For this review, take the finished solid that the model builds, in its own axes (mm). Give positions to 0.01 mm unless a question says otherwise; leave off trailing zeros. Order: outer loops, then holes, each group sorted by start corner. A loop starts at its lowest first (then second) coordinate and runs counter-clockwise, first axis right, second up. Notation, with made-up numbers: (-0.5, 64) - (37.5, 64) arc R29 cw to (37.5, 101) - close; hole circle Ø8 at (9, 18). An arc over 180 degrees is marked (long way). Use a Markdown table: item, result. Add a question column.
1) We need section C-C on y = -23. Write out the cut boundary in (x, z).
2) We need section B-B on x = 0. Write out the cut boundary in (y, z), then the cut area to 3 significant figures.
3) Wall thickness on L1, parallel to Z at x = 0, y = -22; L2, parallel to Z at x = -6, y = -4; L3, parallel to X at y = -4, z = -259.5: over which ranges is each line inside the solid? List them lowest first.
4) We need section A-A on z = 0. Write out the cut boundary in (x, y), then the cut area to 3 significant figures.
5) Clearance check with flat-ended pins moving along their axes: P1, Ø1, axis at y = -21.5, z = 223.5, coming from the -X side; P2, Ø12, axis at x = 161.5, y = -17.5, coming from the -Z side; P3, Ø2, axis at x = 233, y = -39.5, coming from the +Z side. State where each tip first meets the part, or that it passes through.
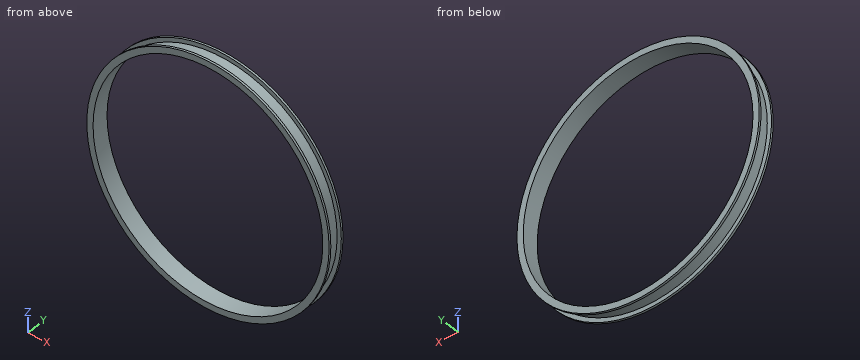
```python
from build123d import *

# Parameters (mm, degrees)
F0_R     = 368.3
F1_DEPTH = 50.8
F2_D     = 698.5
F3_T     = -6.35


with BuildPart() as f1:
    # F0 (on Front) → F1 (new body)
    with BuildSketch(Plane.XZ):
        Circle(F0_R)
    extrude(amount=F1_DEPTH)

    # F2 (through all)
    with Locations(Plane(origin=(0, 0, 0), x_dir=(1, 0, 0), z_dir=(0, 1, 0))):
        with Locations((0, 0)):
            Hole(F2_D / 2)

    # F3
    f3_openings = [f1.faces().sort_by_distance(p)[0] for p in [
        (-368.3, -25.4, 0),
    ]]
    offset(amount=F3_T, openings=f3_openings)


solid = f1.part
```
Checked values:
| question | item | result |
|---|---|---|
| 1 | outline | circle Ø711.2 at (0, 0); hole circle Ø698.5 at (0, 0) |
| 2 | outline | (-50.8, -368.3) - (-44.45, -368.3) - (-44.45, -355.6) - (-6.35, -355.6) - (-6.35, -368.3) - (0, -368.3) - (0, -349.25) - (-50.8, -349.25) - close; (-50.8, 349.25) - (0, 349.25) - (0, 368.3) - (-6.35, 368.3) - (-6.35, 355.6) - (-44.45, 355.6) - (-44.45, 368.3) - (-50.8, 368.3) - close |
| 2 | area | 968 mm² |
| 3 | L1 | -355.6 to -349.25, 349.25 to 355.6 |
| 3 | L2 | -368.25 to -349.2, 349.2 to 368.25 |
| 3 | L3 | -261.35 to -233.74, 233.74 to 261.35 |
| 4 | outline | (-368.3, -50.8) - (-349.25, -50.8) - (-349.25, 0) - (-368.3, 0) - (-368.3, -6.35) - (-355.6, -6.35) - (-355.6, -44.45) - (-368.3, -44.45) - close; (349.25, -50.8) - (368.3, -50.8) - (368.3, -44.45) - (355.6, -44.45) - (355.6, -6.35) - (368.3, -6.35) - (368.3, 0) - (349.25, 0) - close |
| 4 | area | 968 mm² |
| 5 | P1 | x = -276.99 |
| 5 | P2 | z = -319.8 |
| 5 | P3 | z = 269.49 |
